The listing builds one solid part. Answer for the finished solid, in the listing's coordinates (mm). Face numbers are marked on the shaded views. A direction names the side the tool comes from. Give positions to 0.01 mm unless a question says otherwise; leave off trailing zeros. Order: outer loops, then holes, each group sorted by start corner. A loop starts at its lowest first (then second) coordinate and runs counter-clockwise, first axis right, second up.
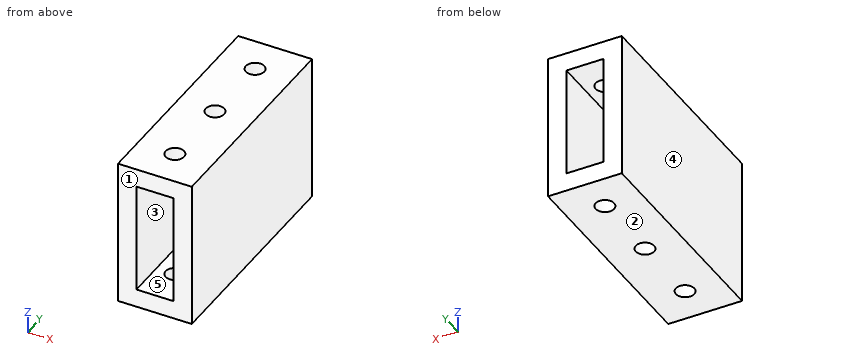
Autodesk Inventor part; units mm, degrees
ref_plane "YZ Plane" through (0, 0, 0) normal (1, 0, 0) x (0, 1, 0)
ref_plane "XZ Plane" through (0, 0, 0) normal (0, 1, 0) x (-1, 0, 0)
ref_plane "XY Plane" through (0, 0, 0) normal (0, 0, 1) x (1, 0, 0)
sketch "Sketch1" plane through (0, 0, 0) normal (0, 0, 1) x (1, 0, 0)
  line L0 (-143.1734, 18.1767) -> (-117.7734, 18.1767)
  line L1 (-117.7734, 18.1767) -> (-117.7734, 94.3767)
  line L2 (-117.7734, 94.3767) -> (-143.1734, 94.3767)
  line L3 (-143.1734, 94.3767) -> (-143.1734, 18.1767)
  point P0 (0, 0)
  dimension "d0" = 76.2
  dimension "d1" = 25.4
extrude "Extrusion1" add sketch "Sketch1" along normal blind 50.8
sketch "Sketch2" plane through (-143.1734, 94.3767, 0) normal (0, 1, 0) x (1, 0, 0)
  line L0 (25.4, 0) -> (0, 0)
  line L1 (0, 0) -> (0, -50.8)
  line L2 (25.4, -50.8) -> (0, -50.8)
  line L3 (25.4, 0) -> (25.4, -50.8)
  line L4 (6.35, -44.45) -> (6.35, -6.35)
  line L5 (6.35, -6.35) -> (19.05, -6.35)
  line L6 (19.05, -6.35) -> (19.05, -44.45)
  line L7 (19.05, -44.45) -> (6.35, -44.45)
  point P0 (143.1734, 0)
  dimension "d4" = 6.35
extrude "Extrusion2" cut sketch "Sketch2" against normal through all contours L4 L5 L6 L7
sketch "Sketch3" plane through (0, 0, 0) normal (0, 0, -1) x (-1, 0, 0)
  line L0 (143.1734, 18.1767) -> (117.7734, 18.1767)
  line L1 (130.4734, 18.1767) -> (130.4734, 94.3767) construction
  line L2 (136.8234, 94.3767) -> (124.1234, 94.3767)
  circle A0 centre (130.4734, 30.8767) radius 3.175
  circle A1 centre (130.4734, 56.2767) radius 3.175
  circle A2 centre (130.4734, 81.6767) radius 3.175
  point P0 (0, 0)
  dimension "d7" = 6.35
  dimension "d8" = 12.7
  dimension "d11" = 25.4
extrude "Extrusion3" cut sketch "Sketch3" against normal through all
properties part number "2AM-17-03-Frame Block"
1) A tool of negligible diameter and unlimited length cuts with its end or side. For the marked faces 4 and 5, from which of +Z, -Z, +X, -X, +Y, -Y can it reach the whole face along a straight path? Write none if from no direction.
Geometry says:
face 4: +Z, -Z, -X, +Y, -Y
face 5: +Y, -Y
2) For a pull along Z with two mould halves and no side action, classify the marked faces 1, 2 and 3 as +Z half, -Z half, draft (parallel to the pull), parting line (faces both ways), or undercut.
Geometry says:
face 1: draft
face 2: -Z half
face 3: undercut
3) Find section C-C (y = 64). Write down the section's boundary in (x, z).
Geometry says:
outline: (-143.17, 0) - (-117.77, 0) - (-117.77, 50.8) - (-143.17, 50.8) - close; hole (-136.82, 6.35) - (-124.12, 6.35) - (-124.12, 44.45) - (-136.82, 44.45) - close
4) Straight lines are drawn through the part: probe 1 along Y at (x, z) = (-130.5, 3.5); probe 2 along X at (y, z) = (35, 34); probe 3 along Z at (x, y) = (-135.75, 55). For each, find the intervals that lie inside material, in ascending order.
Geometry says:
probe 1: y = 18.18 to 27.7, 34.05 to 53.1, 59.45 to 78.5, 84.85 to 94.38
probe 2: x = -143.17 to -136.82, -124.12 to -117.77
probe 3: z = 0 to 6.35, 44.45 to 50.8
5) Find section B-B (z = 31). Write down the section's boundary in (x, y).
Geometry says:
outline: (-143.17, 18.18) - (-136.82, 18.18) - (-136.82, 94.38) - (-143.17, 94.38) - close; (-124.12, 18.18) - (-117.77, 18.18) - (-117.77, 94.38) - (-124.12, 94.38) - close
6) Find section A-A (x = -125). Write down the section's boundary in (y, z).
Geometry says:
outline: (18.18, 0) - (94.38, 0) - (94.38, 6.35) - (18.18, 6.35) - close; (18.18, 44.45) - (94.38, 44.45) - (94.38, 50.8) - (18.18, 50.8) - close
7) Find section D-D (x = -129.25). Count the separate pieces of the cut face and the enclosed holes in it, then the cut area to 3 significant figures.
Geometry says:
separate pieces: 8
enclosed holes: 0
area: 744 mm2
8) Given P1, Ø5, axis at x = -130.47, y = 81.68, coming from the +Z side, flat-ended and moving along its own axis, determine where the tip first touches the part or whether it passes through.
Geometry says:
P1: passes through
